Part model, mm, in its own coordinate system. A direction names the side the tool comes from. Round coordinates to 2 decimals unless told otherwise and drop trailing zeros. Write each loop counter-clockwise with the first axis right and the second up, starting at its lowest first coordinate (ties: lowest second). Pieces come first, ordered by that corner, then holes.
```python
from build123d import *

# Parameters (mm, degrees)
SKETCH_2_R          = 1.35
EXTRUDE_2_DEPTH     = 43
CUT_EXTRUDE_3_DEPTH = 43
SKETCH_6_W          = 4
SKETCH_6_H          = 54
EXTRUDE_3_DEPTH     = 43
SKETCH_7_W          = 2
SKETCH_7_H          = 35
CUT_EXTRUDE_5_DEPTH = 54
SKETCH_8_R          = 1.25
CUT_EXTRUDE_6_DEPTH = 54


with BuildPart() as part:
    # Sketch 2 → Extrude 2 (new body)
    with BuildSketch(Plane.XY):
        with BuildLine():
            Line((-19.925778092, 26.834933958), (-19.925778092, -26.265066042))
            Line((-19.925778092, -26.265066042), (-14.825778092, -32.265066042))
            Line((-14.825778092, -32.265066042), (15.174221908, -32.265066042))
            Line((15.174221908, -32.265066042), (20.274221908, -26.265066042))
            Line((20.274221908, -26.265066042), (20.274221908, 27.734933958))
            Line((20.274221908, 27.734933958), (14.674221908, 32.494933958))
            Line((14.674221908, 32.494933958), (14.674221908, 29.834933958))
            Line((14.674221908, 29.834933958), (14.674221908, -23.665066042))
            ThreePointArc((14.674221908, -23.665066042), (13.795542252, -25.786386386), (11.674221908, -26.665066042))
            Line((11.674221908, -26.665066042), (-11.325778092, -26.665066042))
            ThreePointArc((-11.325778092, -26.665066042), (-13.447098435, -25.786386386), (-14.325778092, -23.665066042))
            Line((-14.325778092, -23.665066042), (-14.325778092, 29.834933958))
            Line((-14.325778092, 29.834933958), (-14.325778092, 32.834933958))
            Line((-14.325778092, 32.834933958), (-14.825778092, 32.834933958))
            Line((-14.825778092, 32.834933958), (-19.925778092, 26.834933958))
        make_face()
        with Locations((17.474221908, -21.665066042)):
            Circle(SKETCH_2_R, mode=Mode.SUBTRACT)
        with Locations((-17.125778092, 22.334933958)):
            Circle(SKETCH_2_R, mode=Mode.SUBTRACT)
        with Locations((-17.125778092, 0.334933958)):
            Circle(SKETCH_2_R, mode=Mode.SUBTRACT)
        with Locations((-17.125778092, -21.665066042)):
            Circle(SKETCH_2_R, mode=Mode.SUBTRACT)
        with Locations((-10.825778092, -29.465066042)):
            Circle(SKETCH_2_R, mode=Mode.SUBTRACT)
        with Locations((11.174221908, -29.465066042)):
            Circle(SKETCH_2_R, mode=Mode.SUBTRACT)
        with Locations((17.474221908, 0.334933958)):
            Circle(SKETCH_2_R, mode=Mode.SUBTRACT)
        with Locations((17.474221908, 22.334933958)):
            Circle(SKETCH_2_R, mode=Mode.SUBTRACT)
    extrude(amount=EXTRUDE_2_DEPTH)

    # Sketch 5 → Cut-Extrude 3 (cut)
    with BuildSketch(Plane(origin=(20.274221908, 0, 0), x_dir=(0, 0, -1), z_dir=(1, 0, 0))):
        Polygon((-39, 32.834933958), (-39, -26.265066042), (-39, -32.265066042), (-4, -32.265066042), (-4, -26.265066042), (-4, 32.834933958), align=None)
    extrude(amount=-CUT_EXTRUDE_3_DEPTH, mode=Mode.SUBTRACT)


with BuildPart() as cut_extrude_3_piece_1:
    # of the separate pieces the step leaves, piece 1, a body of its own (cut_extrude_3_pieces)
    add(part.part.solids().sort_by_distance((-19.925778092, 26.834933958, 39))[0])



with BuildPart() as cut_extrude_3_piece_2:
    # of the separate pieces the step leaves, piece 2, a body of its own (cut_extrude_3_pieces)
    add(part.part.solids().sort_by_distance((-19.925778092, 26.834933958, 0))[0])


with BuildPart() as cut_extrude_3_piece_1_1:
    add(cut_extrude_3_piece_1.part)

    add(cut_extrude_3_piece_2.part)  # Extrude 3 merges Cut-Extrude 3 piece 2
    # Sketch 6 → Extrude 3 (add)
    with BuildSketch(Plane.XY.offset(43)):
        with Locations((22.274221908, 0.734933958)):
            Rectangle(SKETCH_6_W, SKETCH_6_H)
    extrude(amount=-EXTRUDE_3_DEPTH)

    # Sketch 7 → Cut-Extrude 5 (cut)
    with BuildSketch(Plane(origin=(0, 27.734933958, 0), x_dir=(1, 0, 0), z_dir=(0, 1, 0))):
        with Locations((21.274221908, -21.5)):
            Rectangle(SKETCH_7_W, SKETCH_7_H)
    extrude(amount=-CUT_EXTRUDE_5_DEPTH, mode=Mode.SUBTRACT)

    # Sketch 8 → Cut-Extrude 6 (cut)
    with BuildSketch(Plane(origin=(24.274221908, 0, 0), x_dir=(0, 0, -1), z_dir=(1, 0, 0))):
        with Locations(Location((-21.442052439, 0.340563404, 0), (0, 0, 90))):
            Circle(SKETCH_8_R)
        with Locations(Location((-31.442052439, 10.340563404, 0), (0, 0, 90))):
            Circle(SKETCH_8_R)
        with Locations(Location((-11.442052439, 0.340563404, 0), (0, 0, 90))):
            Circle(SKETCH_8_R)
        with Locations(Location((-21.442052439, 10.340563404, 0), (0, 0, 90))):
            Circle(SKETCH_8_R)
        with Locations(Location((-31.442052439, 0.340563404, 0), (0, 0, 90))):
            Circle(SKETCH_8_R)
        with Locations(Location((-11.442052439, 10.340563404, 0), (0, 0, 90))):
            Circle(SKETCH_8_R)
        with Locations(Location((-31.442052439, -9.659436596, 0), (0, 0, 90))):
            Circle(SKETCH_8_R)
        with Locations(Location((-21.442052439, -9.659436596, 0), (0, 0, 90))):
            Circle(SKETCH_8_R)
        with Locations(Location((-11.442052439, -9.659436596, 0), (0, 0, 90))):
            Circle(SKETCH_8_R)
    extrude(amount=-CUT_EXTRUDE_6_DEPTH, mode=Mode.SUBTRACT)


solid = cut_extrude_3_piece_1_1.part
```
Q1. Cut at B-B on y = -5. Write the cut outline in (x, z), plus the area to 3 significant figures.
Values follow:
outline: (-19.93, 0) - (-14.33, 0) - (-14.33, 4) - (-19.93, 4) - close; (-19.93, 39) - (-14.33, 39) - (-14.33, 43) - (-19.93, 43) - close; (14.67, 0) - (24.27, 0) - (24.27, 43) - (14.67, 43) - (14.67, 39) - (22.27, 39) - (22.27, 4) - (14.67, 4) - close
area: 192 mm2
Q2. Cut at D-D on x = -13.5. Write the cut outline in (y, z), plus the area to 3 significant figures.
Values follow:
outline: (-32.27, 0) - (-25.73, 0) - (-25.73, 4) - (-32.27, 4) - close; (-32.27, 39) - (-25.73, 39) - (-25.73, 43) - (-32.27, 43) - close
area: 52.3 mm2
Q3. Cut at A-A on x = -6. Write the cut outline in (y, z), plus the area to 3 significant figures.
Values follow:
outline: (-32.27, 0) - (-26.67, 0) - (-26.67, 4) - (-32.27, 4) - close; (-32.27, 39) - (-26.67, 39) - (-26.67, 43) - (-32.27, 43) - close
area: 44.8 mm2
Q4. Wall check: L1, parallel to X at y = 18.5, z = 41.5; L2, parallel to Z at x = -16, y = 20; L3, parallel to Y at x = 18, z = 2. Give the ranges that are in metal, low to high.
Values follow:
L1: x = -19.93 to -14.33, 14.67 to 24.27
L2: z = 0 to 4, 39 to 43
L3: y = -28.94 to -22.91, -20.42 to -0.91, 1.58 to 21.09, 23.58 to 29.67
Q5. Drop flat-ended pins along their axis: pin 1 (10 mm diameter, centred on y = -8, z = 10, fed in from -X); pin 2 (2 mm diameter, centred on x = -2.5, z = 2.5, fed in from +Y); pin 3 (3 mm diameter, centred on x = 23, z = 19.5, fed in from -Y). Give the stop position or say it passes through.
Values follow:
pin 1: stops at x = 22.27
pin 2: stops at y = -26.67
pin 3: stops at y = -26.27
Q6. Cut at C-C on z = 19. Write the cut outline in (x, y).
Values follow:
outline: (22.27, -26.27) - (24.27, -26.27) - (24.27, 27.73) - (22.27, 27.73) - close
Q7. Mould opens along Y. For faces 1 (the cylindrical face through (23.29, -9.93, 10.22)), 2 (the flat face through (17.689, -29.307, 1.972)), 3 (the flat face through (22.274, 1, 26)), 4 (the cylindrical face through (13.82, -25.76, 1.97)) say: +Y half, -Y half, draft (parallel to the pull), parting line (faces both ways), or undercut.
Values follow:
face 1: undercut
face 2: -Y half
face 3: draft
face 4: +Y half
Q8. Which spindle directions (+Z, -Z, +X, -X, +Y, -Y) get a long thin tool onto all of the face, cutting with end or side? Do faces 5 (the flat face through (0, -26.665, 2)), 6 (the flat face through (17.513, 30.082, 1.972)), 7 (the flat face through (23, -26.265, 22)). Say none if no direction does.
Values follow:
face 5: +Z, -Z, +Y
face 6: +Z, -Z, +X, +Y
face 7: +Z, -Z, +X, -Y
